Check sheet for the modelled part. Datum: model origin and axes. Units: mm. A direction names the side the tool comes from. Round coordinates to 2 decimals unless told otherwise and drop trailing zeros. Order: outer loops, then holes, each group sorted by start corner. A loop starts at its lowest first (then second) coordinate and runs counter-clockwise, first axis right, second up.
Q1. Cross-section at B-B on x = 18. Record the cut outline in (y, z).
Q2. Cross-section at C-C on z = 13.75. Record the cut outline in (x, y).
Q3. Cross-section at A-A on y = -27. Record the cut outline in (x, z), then the cut area to 3 significant figures.
Q4. Set-up check for faces 3 (the cylindrical face through (-33.955, 48.824, 8.874)), 4 (the flat face through (28, 46, 11)): record each of +Z, -Z, +X, -X, +Y, -Y from which the full face is reachable in a straight line by a thin tool's end or side.
Q5. Cross-section at D-D on x = -32. Record the cut outline in (y, z), then the cut area to 3 significant figures.
Q6. Mould release check, pull along X, two halves, no side actions. Record for faces 1 (the flat face through (37, -1, 9)), 2 (the flat face through (19, -51.5, 10)): +X half, -X half, draft (parallel to the pull), parting line (faces both ways), or undercut.
Q7. Scan lines: probe 1 along Y at (x, z) = (-7, 6.5); probe 2 along X at (y, z) = (-25, 7.75); probe 3 along X at (y, z) = (-5.5, 6.5). Record each from-to range of solid material in increasing order.
Q8. Depth check by flat-ended pin: P1, Ø2.5, axis at x = 32.75, y = -6.07, coming from the +Z side; P2, Ø4, axis at x = 19, y = -30.5, coming from the +Z side. Enter the tip coordinate at first touch or a pass-through.
from build123d import *

# Parameters (mm, degrees)
ESQUISSE1_W                          = 74
ESQUISSE1_H                          = 105
BOSS_EXTRU_1_DEPTH                   = 18
ESQUISSE2_W                          = 68
ESQUISSE2_H                          = 99
ENL_V_MAT_EXTRU_1_DEPTH              = 15
ESQUISSE3_W                          = 6
ESQUISSE3_H                          = 6
BOSS_EXTRU_2_DEPTH                   = 15
D_GAGEMENT_M41_D                     = 4.5
ESQUISSE7_W                          = 10
ESQUISSE7_H                          = 30
ENL_V_MAT_EXTRU_2_DEPTH              = 15
R_P_TITION_LIN_AIRE3_COUNT           = 2
R_P_TITION_LIN_AIRE3_PITCH           = 53
R_P_TITION_LIN_AIRE3_COPY_1_SKETCH_W = 6
R_P_TITION_LIN_AIRE3_COPY_1_SKETCH_H = 6
R_P_TITION_LIN_AIRE3_COPY_1_DEPTH    = 15
R_P_TITION_LIN_AIRE3_COPY_2_D        = 4.5
ESQUISSE8_W                          = 68
ESQUISSE8_H                          = 33.530286581
ENL_V_MAT_EXTRU_3_DEPTH              = 2


with BuildPart() as part:
    # Esquisse1 → Boss.-Extru.1 (new body)
    with BuildSketch(Plane.XY):
        Rectangle(ESQUISSE1_W, ESQUISSE1_H)
    extrude(amount=BOSS_EXTRU_1_DEPTH)

    # Esquisse2 → Enlèv. mat.-Extru.1 (cut)
    with BuildSketch(Plane.XY.offset(18)):
        Rectangle(ESQUISSE2_W, ESQUISSE2_H)
    extrude(amount=-ENL_V_MAT_EXTRU_1_DEPTH, mode=Mode.SUBTRACT)

    # Esquisse3 → Boss.-Extru.2 (add)
    with BuildSketch(Plane.XY.offset(18)):
        with Locations((-31, 46.5)):
            Rectangle(ESQUISSE3_W, ESQUISSE3_H)
    boss_extru_2 = extrude(amount=-BOSS_EXTRU_2_DEPTH)

    # Dégagement M41 (through all)
    with Locations(Plane.XY.offset(18)):
        with Locations((-32.745076206, 46.926751476)):
            d_gagement_m41 = Hole(D_GAGEMENT_M41_D / 2)

    # Esquisse7 → Enlèv. mat.-Extru.2 (cut)
    with BuildSketch(Plane.XZ.offset(52.5)):
        with Locations((0, 18)):
            Rectangle(ESQUISSE7_W, ESQUISSE7_H)
    extrude(amount=-ENL_V_MAT_EXTRU_2_DEPTH, mode=Mode.SUBTRACT)

    # Symétrie5: Boss.-Extru.2, Dégagement M41 across plane
    add(boss_extru_2.mirror(Plane(origin=(0, 0, 0), x_dir=(0, 0, 1), z_dir=(1, 0, 0))))
    add(d_gagement_m41.mirror(Plane(origin=(0, 0, 0), x_dir=(0, 0, 1), z_dir=(1, 0, 0))), mode=Mode.SUBTRACT)

    # Répétition linéaire3: Boss.-Extru.2, Dégagement M41 ×2
    with Locations(*[(0, -i * R_P_TITION_LIN_AIRE3_PITCH, 0) for i in range(1, R_P_TITION_LIN_AIRE3_COUNT)]):
        add(boss_extru_2)
        add(d_gagement_m41, mode=Mode.SUBTRACT)

    # Répétition linéaire3 copy 1 sketch → Répétition linéaire3 copy 1 (add)
    with BuildSketch(Plane(origin=(0, -53, 18), x_dir=(-1, 0, 0), z_dir=(0, 0, 1))):
        with Locations((-31, -46.5)):
            Rectangle(R_P_TITION_LIN_AIRE3_COPY_1_SKETCH_W, R_P_TITION_LIN_AIRE3_COPY_1_SKETCH_H)
    extrude(amount=-R_P_TITION_LIN_AIRE3_COPY_1_DEPTH)

    # Répétition linéaire3 copy 2 (through all)
    with Locations(Plane(origin=(0, -53, 18), x_dir=(-1, 0, 0), z_dir=(0, 0, 1))):
        with Locations((-32.745076206, -46.926751476)):
            Hole(R_P_TITION_LIN_AIRE3_COPY_2_D / 2)

    # Esquisse8 → Enlèv. mat.-Extru.3 (cut)
    with BuildSketch(Plane(origin=(0, -49.5, 0), x_dir=(1, 0, 0), z_dir=(0, 1, 0))):
        with Locations((0, -19.765143291)):
            Rectangle(ESQUISSE8_W, ESQUISSE8_H)
    extrude(amount=-ENL_V_MAT_EXTRU_3_DEPTH, mode=Mode.SUBTRACT)


solid = part.part
Results found:
1. outline: (-52.5, 0) - (52.5, 0) - (52.5, 18) - (49.5, 18) - (49.5, 3) - (-51.5, 3) - (-51.5, 18) - (-52.5, 18) - close
2. outline: (-37, -52.5) - (-5, -52.5) - (-5, -51.5) - (-34, -51.5) - (-34, -9.5) - (-28, -9.5) - (-28, -3.5) - (-34, -3.5) - (-34, 43.5) - (-28, 43.5) - (-28, 49.5) - (28, 49.5) - (28, 43.5) - (34, 43.5) - (34, -3.5) - (28, -3.5) - (28, -9.5) - (34, -9.5) - (34, -51.5) - (5, -51.5) - (5, -52.5) - (37, -52.5) - (37, 52.5) - (-37, 52.5) - close; hole circle Ø4.5 at (-32.75, -6.07); hole circle Ø4.5 at (-32.75, 46.93); hole circle Ø4.5 at (32.75, -6.07); hole circle Ø4.5 at (32.75, 46.93)
3. outline: (-37, 0) - (37, 0) - (37, 18) - (34, 18) - (34, 3) - (-34, 3) - (-34, 18) - (-37, 18) - close
3. area: 312 mm2
4. face 3: +Z, -Z
4. face 4: +Z
5. outline: (-52.5, 0) - (-8.2, 0) - (-8.2, 18) - (-9.5, 18) - (-9.5, 3) - (-51.5, 3) - (-51.5, 18) - (-52.5, 18) - close; (-3.95, 0) - (44.8, 0) - (44.8, 18) - (43.5, 18) - (43.5, 3) - (-3.5, 3) - (-3.5, 18) - (-3.95, 18) - close; (49.05, 0) - (52.5, 0) - (52.5, 18) - (49.05, 18) - close
5. area: 402 mm2
6. face 1: +X half
6. face 2: undercut
7. probe 1: y = -52.5 to -51.5, 49.5 to 52.5
7. probe 2: x = -37 to -34, 34 to 37
7. probe 3: x = -37 to -34.92, -30.57 to -28, 28 to 30.57, 34.92 to 37
8. P1: passes through
8. P2: stops at z = 3
